Part model, mm, in its own coordinate system. Coordinates: 2 decimals unless noted, no trailing zeros. Order: outer loops, then holes, each group sorted by start corner. A loop starts at its lowest first (then second) coordinate and runs counter-clockwise, first axis right, second up. Notation, with made-up numbers: M 84,48 L 127,48 A17 cw 127,73 Z; hole C 71.5,-18.75 d9. An arc over 180 degrees is marked long. Write item = value, one per line. Start each with the question number.
from build123d import *

# Parameters (mm, degrees)
RESSALTO_EXTRUS_O1_DEPTH = 3


with BuildPart() as part:
    # Esboço1 → Ressalto-extrusão1 (new body)
    with BuildSketch(Plane.XY):
        with BuildLine():
            Line((46.5, -1.5), (46.5, -0.5))
            Line((46.5, -0.5), (52.5, -0.5))
            ThreePointArc((52.5, -0.5), (58.156854249, 1.843145751), (60.5, 7.5))
            Line((60.5, 7.5), (60.5, 38.5))
            ThreePointArc((60.5, 38.5), (58.156854249, 44.156854249), (52.5, 46.5))
            Line((52.5, 46.5), (46.5, 46.5))
            Line((46.5, 46.5), (46.5, 47.5))
            ThreePointArc((46.5, 47.5), (44.156854249, 53.156854249), (38.5, 55.5))
            Line((38.5, 55.5), (7.5, 55.5))
            ThreePointArc((7.5, 55.5), (1.843145751, 53.156854249), (-0.5, 47.5))
            Line((-0.5, 47.5), (-0.5, 46.5))
            Line((-0.5, 46.5), (-1.5, 46.5))
            ThreePointArc((-1.5, 46.5), (-7.156854249, 44.156854249), (-9.5, 38.5))
            Line((-9.5, 38.5), (-9.5, 7.5))
            ThreePointArc((-9.5, 7.5), (-7.156854249, 1.843145751), (-1.5, -0.5))
            Line((-1.5, -0.5), (-0.5, -0.5))
            Line((-0.5, -0.5), (-0.5, -1.5))
            ThreePointArc((-0.5, -1.5), (1.843145751, -7.156854249), (7.5, -9.5))
            Line((7.5, -9.5), (38.5, -9.5))
            ThreePointArc((38.5, -9.5), (44.156854249, -7.156854249), (46.5, -1.5))
        make_face()
        with BuildLine():
            Line((41.5, -1.5), (41.5, 0))
            ThreePointArc((41.5, 0), (42.818019485, 3.181980515), (46, 4.5))
            Line((46, 4.5), (52.5, 4.5))
            ThreePointArc((52.5, 4.5), (54.621320344, 5.378679656), (55.5, 7.5))
            Line((55.5, 7.5), (55.5, 38.5))
            ThreePointArc((55.5, 38.5), (54.621320344, 40.621320344), (52.5, 41.5))
            Line((52.5, 41.5), (46, 41.5))
            ThreePointArc((46, 41.5), (42.818019485, 42.818019485), (41.5, 46))
            Line((41.5, 46), (41.5, 47.5))
            ThreePointArc((41.5, 47.5), (40.621320344, 49.621320344), (38.5, 50.5))
            Line((38.5, 50.5), (7.5, 50.5))
            ThreePointArc((7.5, 50.5), (5.378679656, 49.621320344), (4.5, 47.5))
            Line((4.5, 47.5), (4.5, 46))
            ThreePointArc((4.5, 46), (3.181980515, 42.818019485), (0, 41.5))
            Line((0, 41.5), (-1.5, 41.5))
            ThreePointArc((-1.5, 41.5), (-3.621320344, 40.621320344), (-4.5, 38.5))
            Line((-4.5, 38.5), (-4.5, 7.5))
            ThreePointArc((-4.5, 7.5), (-3.621320344, 5.378679656), (-1.5, 4.5))
            Line((-1.5, 4.5), (0, 4.5))
            ThreePointArc((0, 4.5), (3.181980515, 3.181980515), (4.5, 0))
            Line((4.5, 0), (4.5, -1.5))
            ThreePointArc((4.5, -1.5), (5.378679656, -3.621320344), (7.5, -4.5))
            Line((7.5, -4.5), (38.5, -4.5))
            ThreePointArc((38.5, -4.5), (40.621320344, -3.621320344), (41.5, -1.5))
        make_face(mode=Mode.SUBTRACT)
    extrude(amount=RESSALTO_EXTRUS_O1_DEPTH)


solid = part.part
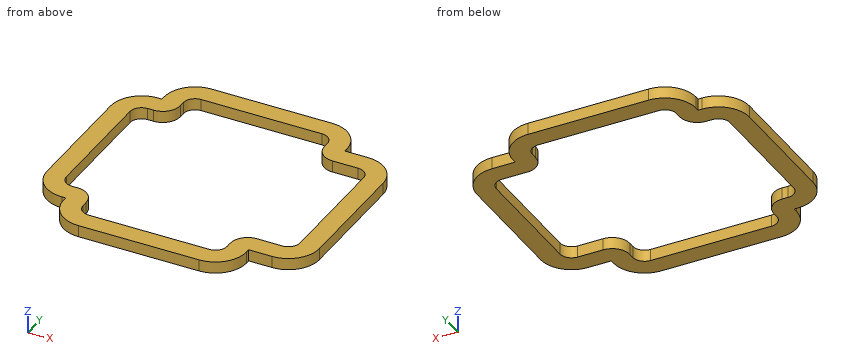
Item 1: Flat gauge pins, fed straight in: pin 1 (0.8 mm diameter, centred on x = -1, z = 1.5, fed in from -Y); pin 2 (0.5 mm diameter, centred on y = -1, z = 1, fed in from +X); pin 3 (0.5 mm diameter, centred on x = -1, z = 1.5, fed in from +Y); pin 4 (2 mm diameter, centred on x = 45.5, y = 44, fed in from -Z). Where does each tip first touch, or does it go through?
Item 2: Cut at B-B, the plane x = 23. Write the cut outline in (y, z).
Item 3: Wall check: line 1 along X through (y, z) = (13, 0.45); line 2 along Y through (x, z) = (47, 2.75); line 3 along Y through (x, z) = (34.5, 2.1). Give the ranges that are in metal, low to high. Write a range as [from, to].
Item 4: Cut at A-A, the plane y = 28.5. Write the cut outline in (x, z).
Filled sheet:
q1.pin_1 = -0.5
q1.pin_2 = 46.5
q1.pin_3 = 46.5
q1.pin_4 = 0
q2.outline = M -9.5,0 L -4.5,0 L -4.5,3 L -9.5,3 Z; M 50.5,0 L 55.5,0 L 55.5,3 L 50.5,3 Z
q3.line_1 = [-9.5, -4.5], [55.5, 60.5]
q3.line_2 = [-0.5, 4.5], [41.5, 46.5]
q3.line_3 = [-9.5, -4.5], [50.5, 55.5]
q4.outline = M -9.5,0 L -4.5,0 L -4.5,3 L -9.5,3 Z; M 55.5,0 L 60.5,0 L 60.5,3 L 55.5,3 Z
